Geometry check sheet. Reference: the model listing, model coordinates, mm. A direction names the side the tool comes from. Give positions to 0.01 mm unless a question says otherwise; leave off trailing zeros. Write each loop counter-clockwise with the first axis right and the second up, starting at its lowest first coordinate (ties: lowest second). Pieces come first, ordered by that corner, then holes. Notation, with made-up numbers: (-34, 76) -> (-6, 76) arc R21 ccw to (-6, 82) -> close; hole circle Ø10 at (37, 60.5). An arc over 180 degrees is marked (long way). One line per item, written item: value.
from build123d import *

# Parameters (mm, degrees)
F0_R     = 44.45
F0_R_2   = 6.35
F1_DEPTH = 12.7
F2_R     = 12.69999
F4_DEPTH = 12.7


# Not quite as in the source:
# - a fillet or chamfer is up to 0.001 mm smaller than in the source, because OpenCascade refuses the exact size


with BuildPart() as f1:
    # F0 (on Right) → F1 (new body, symmetric)
    with BuildSketch(Plane.YZ):
        Circle(F0_R)
        Circle(F0_R_2, mode=Mode.SUBTRACT)
    extrude(amount=F1_DEPTH, both=True)

    # F2 (radius 12.7 in the source; OpenCascade refuses exactly that, so slightly less here)
    f2_edges = [f1.edges().sort_by_distance(p)[0] for p in [
        (12.7, -44.45, 0),
        (-12.7, -44.45, 0),
    ]]
    fillet(f2_edges, radius=F2_R)

    # F3 (on Front) → F4 (join, symmetric)
    with BuildSketch(Plane.XZ):
        Polygon((15.875, 63.5), (-15.875, 63.5), (-15.875, 12.7), (-15.875, -12.7), (15.875, -12.7), (15.875, 12.7), align=None)
    extrude(amount=F4_DEPTH, both=True)


solid = f1.part
1) Sectioned sample at C-C on x = 6. Record the cut outline in (y, z), plus the area to 3 significant figures.
Verdict:
outline: (-12.7, 41.02) arc R42.94 ccw (long way) to (12.7, 41.02) -> (12.7, 63.5) -> (-12.7, 63.5) -> close
area: 6,330 mm^2
2) Sectioned sample at D-D on x = -11. Record the cut outline in (y, z), plus the area to 3 significant figures.
Verdict:
outline: (-12.7, 35.92) arc R38.1 ccw (long way) to (12.7, 35.92) -> (12.7, 63.5) -> (-12.7, 63.5) -> close
area: 5,220 mm^2
3) Tool access check on faces 1 (the flat face through (0, -12.7, 43)), 2 (the flat face through (14, 0, -12.7)), 3 (the flat face through (-14, 0, -12.7)), 4 (the flat face through (0, 12.7, 43)). Record the directions out of +Z, -Z, +X, -X, +Y, -Y that give a thin tool (end or side, any length) a straight path to the whole face; none if there is none.
Verdict:
face 1: +Z, -Y
face 2: -Z, +X, +Y, -Y
face 3: -Z, -X, +Y, -Y
face 4: +Z, +Y
4) Scan lines: probe 1 along X at (y, z) = (25, -20); probe 2 along Z at (x, y) = (13, -11.5). Record each from-to range of solid material in increasing order.
Verdict:
probe 1: -12.7 to 12.7
probe 2: -12.7 to 63.5
5) Depth check by flat-ended pin: pin 1 Ø3.5 at (x, y) = (14.5, 5) entering from -Z; pin 2 Ø6 at (y, z) = (10, -17.5) entering from +X; pin 3 Ø1 at (x, z) = (0, 14) entering from +Y. Enter the tip coordinate at first touch or a pass-through.
Verdict:
pin 1: z = -12.7
pin 2: x = 12.7
pin 3: y = 42.35
